Read the model definition and answer for the solid it produces. Units are mm, in the model's axes. Round coordinates to 2 decimals unless told otherwise and drop trailing zeros. Loops run counter-clockwise (first coordinate to the right, second up) from the corner with the lowest first, then second, coordinate; pieces in that order, holes last. Notation, with made-up numbers: M 11,76 L 69,76 A4 ccw 69,80 Z; hole C 87.25,19.5 d8. An arc over 180 degrees is marked long. Answer as CSV lines item,"result".
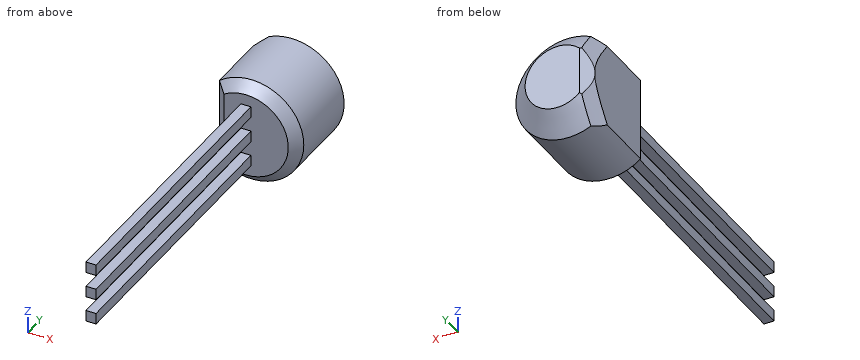
Autodesk Inventor part; units mm, degrees
ref_plane "YZ Plane" through (0, 0, 0) normal (1, 0, 0) x (0, 1, 0)
ref_plane "XZ Plane" through (0, 0, 0) normal (0, 1, 0) x (-1, 0, 0)
ref_plane "XY Plane" through (0, 0, 0) normal (0, 0, 1) x (1, 0, 0)
sketch "Sketch1" plane through (0, 0, 0) normal (0, 1, 0) x (-1, 0, 0)
  circle A0 centre (0, 0) radius 2.6
  line L0 (1.59, 2.0572) -> (1.59, -2.0572)
  dimension "d0" = 5.2
  dimension "d1" = 4.19
extrude "Extrusion1" add sketch "Sketch1" along normal blind 5.2 contours L0 A0 picked at (-1.6247, 0.0943)
sketch "Sketch2" plane through (0, 0, 0) normal (1, 0, 0) x (0, 1, 0)
  line L0 (0, 1.545) -> (-14.2, 1.545)
  line L1 (-14.2, 1.545) -> (-14.2, 0.995)
  line L2 (-14.2, 0.995) -> (0, 0.995)
  line L3 (0, 0.995) -> (0, 1.545)
  line L4 (0, 0.275) -> (-14.2, 0.275)
  line L5 (-14.2, 0.275) -> (-14.2, -0.275)
  line L6 (-14.2, -0.275) -> (0, -0.275)
  line L7 (0, -0.275) -> (0, 0.275)
  line L8 (0, -1.545) -> (-14.2, -1.545)
  line L9 (-14.2, -1.545) -> (-14.2, -0.995)
  line L10 (-14.2, -0.995) -> (0, -0.995)
  line L11 (0, -0.995) -> (0, -1.545)
  line L12 (0, -2.6) -> (0, 2.6)
  point P0 (0, 0)
  point P1 (0, 2.0572)
  point P2 (0, -2.0572)
  dimension "d4" = 14.2
  dimension "d5" = 14.2
  dimension "d6" = 14.2
  dimension "d7" = 0
  dimension "d8" = 0
  dimension "d9" = 0.55
  dimension "d10" = 0.55
  dimension "d11" = 0.55
  dimension "d12" = 0.275
  dimension "d13" = 0.995
  dimension "d14" = 0.995
extrude "Extrusion2" add sketch "Sketch2" along normal mid plane 0.5
chamfer "Chamfer1" distance 1 angle 45 1 edges at (2.6, 5.2, 0)
chamfer "Chamfer2" distance 0.5 angle 45 1 edges at (2.6, 0, 0)
chamfer "Chamfer3" distance 0.5 angle 45 3 edges at (-1.59, 4.9218, -0.9998) (-1.59, 4.9218, 0.9998) (-1.59, 5.2, 0)
chamfer "Chamfer4" distance 0.5 angle 45 1 edges at (-1.59, 0, 0)
properties part number "LM35CAZ"
1) Each of these flat-tipped pins is pushed along its axis until it touches: P1, Ø0.6, axis at y = -8.5, z = 0, coming from the -X side; P2, Ø1.5, axis at y = -1, z = -2, coming from the +X side; P3, Ø0.6, axis at x = 0, y = -5.5, coming from the +Z side (3 decimals); P4, Ø2, axis at y = 1, z = 1, coming from the +X side. Where does it stop, or does it pass through?
Evaluation:
P1,"stops at x = -0.25"
P2,"stops at x = 0.25"
P3,"stops at z = 1.545"
P4,"stops at x = 2.6"
2) Find section B-B, the plane x = 0. Give the vertices of the cut face in (y, z) (3 decimals), then the cut area to 3 significant figures.
Evaluation:
outline,"M -14.2,-1.545 L 0,-1.545 L 0,-2.1 L 0.5,-2.6 L 4.2,-2.6 L 5.2,-1.6 L 5.2,1.6 L 4.2,2.6 L 0.5,2.6 L 0,2.1 L 0,1.545 L -14.2,1.545 L -14.2,0.995 L 0,0.995 L 0,0.275 L -14.2,0.275 L -14.2,-0.275 L 0,-0.275 L 0,-0.995 L -14.2,-0.995 Z"
area,"49.2 mm^2"
3) Straight lines are drawn through the part: line 1 (Z direction, x = -0.05, y = -2.75) (3 decimals); line 2 (Y direction, x = 0.15, z = 0.55); line 3 (X direction, y = 2.25, z = 0.1). For each, find the intervals that lie inside material, in ascending order.
Evaluation:
line 1,"z = -1.545 to -0.995, -0.275 to 0.275, 0.995 to 1.545"
line 2,"y = 0 to 5.2"
line 3,"x = -1.59 to 2.6"
4) Find section A-A, the plane y = -12.5. Give the vertices of the cut face in (x, z) (3 decimals).
Evaluation:
outline,"M -0.25,-1.545 L 0.25,-1.545 L 0.25,-0.995 L -0.25,-0.995 Z; M -0.25,-0.275 L 0.25,-0.275 L 0.25,0.275 L -0.25,0.275 Z; M -0.25,0.995 L 0.25,0.995 L 0.25,1.545 L -0.25,1.545 Z"
5) Find section C-C, the plane y = 2. Give the vertices of the cut face in (x, z).
Evaluation:
outline,"M -1.59,-2.06 A2.6 ccw long -1.59,2.06 Z"
